Verification items for this drawing (mm, ordinates from the low corner). A direction names the side the tool comes from. Round coordinates to 2 decimals unless told otherwise and drop trailing zeros. Write each loop counter-clockwise with the first axis right and the second up, starting at its lowest first coordinate (ties: lowest second). Pieces come first, ordered by that corner, then holes. Notation, with made-up numbers: M -34,80 L -1,80 A10 cw -1,90 Z; hole C -14.75,-31.75 d9. An arc over 180 degrees is marked long. Write each question's results on one line, items separated by ' | '.
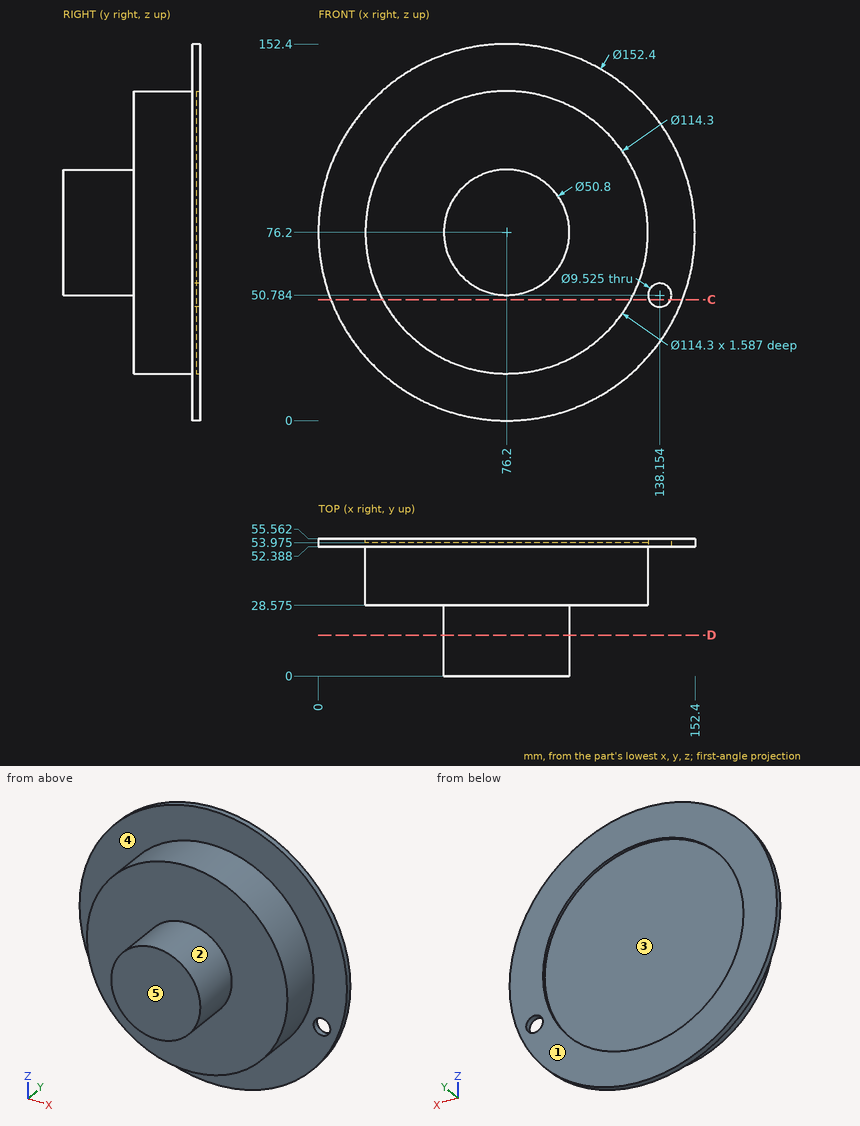
1) Draft check along X on the marked faces 1, 2 and 3. Enter one of: pulls with the +X half, pulls with the -X half, needs draft (parallel to the pull), parting line crosses it, or undercut.
Calculated:
face 1: needs draft | face 2: parting line crosses it | face 3: undercut
2) Material ranges on line 1 (Z direction, x = 76.2, y = 54.6); line 2 (Y direction, x = 145, z = 65); line 3 (Y direction, x = 79.5, z = 121.5) (1 decimal), recorded low to high. Write a range as [from, to].
Calculated:
line 1: z = [0, 19.05], [133.35, 152.4] | line 2: y = [52.39, 55.56] | line 3: y = [28.6, 54]
3) Access from +Z, -Z, +X, -X, +Y, -Y to the whole of each face (thin tool, end or side, straight path). Record for the marked faces 4 and 5.
Calculated:
face 4: -Y | face 5: +Z, -Z, +X, -X, -Y
4) Depth check by flat-ended pin: P1, Ø12.5, axis at x = 138.15, z = 50.78, coming from the +Y side; P2, Ø1.5, axis at x = 52, y = 19, coming from the -Z side; P3, Ø3, axis at x = 76.5, y = 25.5, coming from the -Z side; P4, Ø8, axis at x = 46, z = 116, coming from the +Y side (1 decimal). Enter the tip coordinate at first touch or a pass-through.
Calculated:
P1: stops at y = 55.56 | P2: stops at z = 66.44 | P3: stops at z = 50.8 | P4: stops at y = 54
5) Sectioned sample at D-D, the plane y = 16.5. Record the cut outline in (x, z).
Calculated:
outline: C 76.2,76.2 d50.8
6) Sectioned sample at C-C, the plane z = 49. Record the cut outline in (x, y) (1 decimal), and give its area (3 significant figures).
Calculated:
outline: M 5,52.4 L 25.9,52.4 L 25.9,28.6 L 126.5,28.6 L 126.5,52.4 L 133.7,52.4 L 133.7,55.6 L 126.5,55.6 L 126.5,54 L 25.9,54 L 25.9,55.6 L 5,55.6 Z; M 142.6,52.4 L 147.4,52.4 L 147.4,55.6 L 142.6,55.6 Z | area: 2,660 mm²
